The listing builds one solid part. Answer for the finished solid, in the listing's coordinates (mm). Give positions to 0.01 mm unless a question says otherwise; leave off trailing zeros. Order: outer loops, then holes, each group sorted by start corner. A loop starts at its lowest first (then second) coordinate and runs counter-clockwise, first axis right, second up. Notation, with made-up numbers: (15, 2) - (33, 2) arc R11 ccw to (33, 16) - close; hole circle Ø1 at (21.5, -4). An arc over 180 degrees is marked (long way). Answer in a Markdown table with one row per item.
from build123d import *

# Parameters (mm, degrees)
F0_W     = 180
F0_H     = 120
F0_R     = 5.75
F0_W_2   = 100
F0_H_2   = 60.4
F1_DEPTH = 6
F2_R     = 10


with BuildPart() as f1:
    # F0 (on Front) → F1 (new body)
    with BuildSketch(Plane.XZ):
        Rectangle(F0_W, F0_H)
        with Locations((-75, -45)):
            Circle(F0_R, mode=Mode.SUBTRACT)
        with Locations((75, -45)):
            Circle(F0_R, mode=Mode.SUBTRACT)
        with Locations((-75, 45)):
            Circle(F0_R, mode=Mode.SUBTRACT)
        Rectangle(F0_W_2, F0_H_2, mode=Mode.SUBTRACT)
        with Locations((75, 45)):
            Circle(F0_R, mode=Mode.SUBTRACT)
    extrude(amount=F1_DEPTH)

    # F2
    f2_edges = [f1.edges().sort_by_distance(p)[0] for p in [
        (-90, -3, 60),
        (90, -3, 60),
        (90, -3, -60),
        (-90, -3, -60),
    ]]
    fillet(f2_edges, radius=F2_R)


solid = f1.part
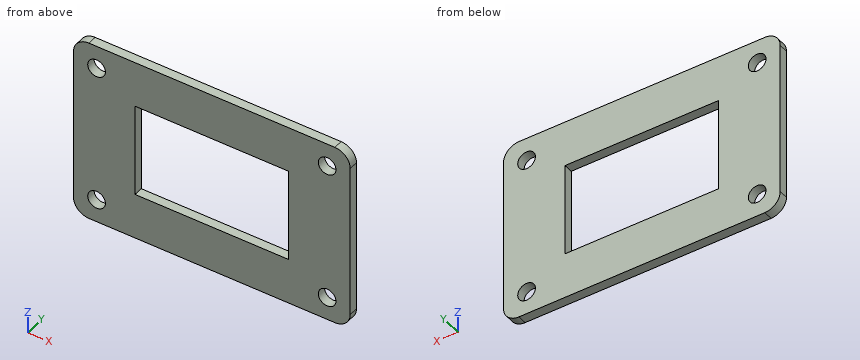
Item 1: This flat-tipped pin is pushed along its axis until it touches: P1, Ø7, axis at x = 75, z = -45, coming from the -Y side. Where does it stop, or does it pass through?
Answer block:
| item | result |
|---|---|
| P1 | through |
Item 2: Find section D-D on y = -5.1. Write down the section's boundary in (x, z), then the cut area to 3 significant figures.
Answer block:
| item | result |
|---|---|
| outline | (-90, -50) arc R10 ccw to (-80, -60) - (80, -60) arc R10 ccw to (90, -50) - (90, 50) arc R10 ccw to (80, 60) - (-80, 60) arc R10 ccw to (-90, 50) - close; hole circle Ø11.5 at (-75, -45); hole circle Ø11.5 at (-75, 45); hole (-50, -30.2) - (50, -30.2) - (50, 30.2) - (-50, 30.2) - close; hole circle Ø11.5 at (75, -45); hole circle Ø11.5 at (75, 45) |
| area | 15,100 mm² |
Item 3: Find section B-B on z = -1.5. Write down the section's boundary in (x, y), then the cut area to 3 significant figures.
Answer block:
| item | result |
|---|---|
| outline | (-90, -6) - (-50, -6) - (-50, 0) - (-90, 0) - close; (50, -6) - (90, -6) - (90, 0) - (50, 0) - close |
| area | 480 mm² |
Item 4: Find section A-A on x = 16. Write down the section's boundary in (y, z), then the cut area to 3 significant figures.
Answer block:
| item | result |
|---|---|
| outline | (-6, -60) - (0, -60) - (0, -30.2) - (-6, -30.2) - close; (-6, 30.2) - (0, 30.2) - (0, 60) - (-6, 60) - close |
| area | 358 mm² |
Item 5: Find section C-C on z = -45. Write down the section's boundary in (x, y), then the cut area to 3 significant figures.
Answer block:
| item | result |
|---|---|
| outline | (-90, -6) - (-80.75, -6) - (-80.75, 0) - (-90, 0) - close; (-69.25, -6) - (69.25, -6) - (69.25, 0) - (-69.25, 0) - close; (80.75, -6) - (90, -6) - (90, 0) - (80.75, 0) - close |
| area | 942 mm² |
Item 6: Consider line 1 (Z direction, x = 75, y = -2.65); line 2 (Z direction, x = 33, y = -3.6); line 3 (X direction, y = -3.7, z = -8.5). Determine where each line is inside the solid, lowest interval first.
Answer block:
| item | result |
|---|---|
| line 1 | -60 to -50.75, -39.25 to 39.25, 50.75 to 60 |
| line 2 | -60 to -30.2, 30.2 to 60 |
| line 3 | -90 to -50, 50 to 90 |
